Source: CAD feature listing. Evaluate the final solid. Frame: model axes, mm. A direction names the side the tool comes from. Give positions to 0.01 mm unless a question says otherwise; leave off trailing zeros. Order: outer loops, then holes, each group sorted by start corner. A loop starts at its lowest first (then second) coordinate and runs counter-clockwise, first axis right, second up. Notation, with made-up numbers: M -35,21.5 L -1,21.5 A19 ccw -1,52.5 Z; hole C 7.25,53.5 d3. An arc over 180 degrees is marked long. Answer in a Markdown table with one row per item. Add a question column.
(1) Material intervals for line 1 along Z through (x, y) = (0, 51); line 2 along X through (y, z) = (39, 0), sorted ascending.
(2) Section query A-A, the plane x = 0. Return loops of the section in (y, z).
(3) Section query B-B, the plane z = 0. Return loops of the section in (x, y), plus the area to 3 significant figures.
(4) Set-up query: faces 1 (the face through (203.61, 47.745, 391.465)), 2 (the face through (463.796, 54.86, -146.056)). Return all of +Z, -Z, +X, -X, +Y, -Y with unobstructed straight access to the full face (end or side cutting, diameter ignored); none if empty.
(5) Mould query, pull axis Z, two halves, no side actions, for faces 3 (the face through (-1, 85, -1)), 4 (the face through (-6, 30, -104)), 5 (the face through (-467.89, 19.01, 103.9)). Classes: pulls with the +Z half, pulls with the -Z half, needs draft (parallel to the pull), parting line crosses it, or undercut.
(6) Pin query (flat end, axial travel): P1, Ø1.5, axis at y = 36, z = 28, coming from the +X side; P2, Ø12, axis at x = -111, y = 60, coming from the -Z side; P3, Ø12, axis at y = 53, z = -151, coming from the +X side. Return the tip coordinate at first contact, or that it passes through.
from build123d import *

# Parameters (mm, degrees)
SKETCH1_R           = 486.25
BOSS_EXTRUDE1_DEPTH = 65
SKETCH3_R           = 441.25
CUT_EXTRUDE1_DEPTH  = 35
SKETCH6_R           = 100
BOSS_EXTRUDE3_DEPTH = 55


with BuildPart() as part:
    # Sketch1 → Boss-Extrude1 (new body)
    with BuildSketch(Plane(origin=(0, 0, 0), x_dir=(1, 0, 0), z_dir=(0, 1, 0))):
        Circle(SKETCH1_R)
    extrude(amount=BOSS_EXTRUDE1_DEPTH)

    # Sketch3 → Cut-Extrude1 (cut)
    with BuildSketch(Plane(origin=(0, 65, 0), x_dir=(1, 0, 0), z_dir=(0, 1, 0))):
        Circle(SKETCH3_R)
    extrude(amount=-CUT_EXTRUDE1_DEPTH, mode=Mode.SUBTRACT)

    # Sketch5 → Cut-Revolve1 (revolve, cut)
    with BuildSketch(Plane(origin=(0, 0, 0), x_dir=(0, 0, -1), z_dir=(1, 0, 0))):
        Polygon((486.25, 45), (478.929491924, 17.679491924), (461.25, 0), (486.25, 0), align=None)
    revolve(axis=Axis((0, 89.25, 0), (0, -1, 0)), mode=Mode.SUBTRACT)

    # Sketch6 → Boss-Extrude3 (add)
    with BuildSketch(Plane(origin=(0, 30, 0), x_dir=(1, 0, 0), z_dir=(0, 1, 0))):
        Circle(SKETCH6_R)
    extrude(amount=BOSS_EXTRUDE3_DEPTH)


solid = part.part
Values follow:
| question | item | result |
|---|---|---|
| 1 | line 1 | z = -486.25 to -441.25, -100 to 100, 441.25 to 486.25 |
| 1 | line 2 | x = -484.64 to -441.25, -100 to 100, 441.25 to 484.64 |
| 2 | outline | M 0,-461.25 L 17.68,-478.93 L 45,-486.25 L 65,-486.25 L 65,-441.25 L 30,-441.25 L 30,-100 L 85,-100 L 85,100 L 30,100 L 30,441.25 L 65,441.25 L 65,486.25 L 45,486.25 L 17.68,478.93 L 0,461.25 Z |
| 3 | outline | M -486.25,45 L -478.93,17.68 L -461.25,0 L 461.25,0 L 478.93,17.68 L 486.25,45 L 486.25,65 L 441.25,65 L 441.25,30 L 100,30 L 100,85 L -100,85 L -100,30 L -441.25,30 L -441.25,65 L -486.25,65 Z |
| 3 | area | 42,600 mm² |
| 4 | face 1 | +Y |
| 4 | face 2 | +Y, -Y |
| 5 | face 3 | needs draft |
| 5 | face 4 | undercut |
| 5 | face 5 | parting line crosses it |
| 6 | P1 | stops at x = 483.23 |
| 6 | P2 | stops at z = -474.78 |
| 6 | P3 | stops at x = 464.13 |
